from build123d import *

# Parameters (mm, degrees)
F2_R     = 2
F3_DEPTH = 1.1
F4_R     = 2.5
F5_DEPTH = 30


with BuildPart() as f1:
    # F0 (on Front) → F1 (revolve)
    with BuildSketch(Plane.XZ):
        Polygon((0, 1.9), (0, 0), (2.45, 1.9), align=None)
    revolve(axis=Axis((0, 0, 0.95), (0, 0, 1)))

    # F2 (on face) → F3 (join)
    with BuildSketch(Plane.XY.offset(1.9)):
        Circle(F2_R)
    extrude(amount=F3_DEPTH)

    # F4 (on face) → F5 (join)
    with BuildSketch(Plane.XY.offset(3)):
        with Locations((0, -0.214779)):
            Circle(F4_R)
    extrude(amount=F5_DEPTH)


solid = f1.part
The model under review builds one solid part; all positions refer to its coordinate system, in mm. A direction names the side the tool comes from. Give positions to 0.01 mm unless a question says otherwise; leave off trailing zeros. Write each loop counter-clockwise with the first axis right and the second up, starting at its lowest first coordinate (ties: lowest second). Pieces come first, ordered by that corner, then holes.
1. For P1, Ø1, axis at y = 1.5, z = 19, coming from the +X side (3 decimals); P2, Ø2, axis at x = 0, y = -1.5, coming from the -Z side, all flat-tipped, find the tip position at first contact; note any pin that passes through.
2. Tool access review of faces 1 (the cylindrical face through (-0.542, -2.655, 17.79)), 2 (the cylindrical face through (-0.434, -1.952, 2.442)): name each direction out of +Z, -Z, +X, -X, +Y, -Y from which nothing blocks a thin tool from reaching the whole face with its end or side.
3. Draft analysis for pull direction Z (two halves, no side actions). For faces 3 (the flat face through (1, -2, 3)), 4 (the conical face through (0, 0, 0)), 5 (the flat face through (0, 0, 33)), state which applies: +Z half, -Z half, draft (parallel to the pull), parting line (faces both ways), or undercut.
4. Wall thickness on L1, parallel to Z at x = -1.6, y = -1.55; L2, parallel to X at y = -0.7, z = 21.5; L3, parallel to X at y = 1.7, z = 11: over which ranges is each line inside the solid? List them lowest first.
5. Add section A-A, the plane z = 19. Write out the cut boundary in (x, y).
Worked answers:
1. P1: stops at x = 2.185
1. P2: stops at z = 0.39
2. face 1: +Z
2. face 2: none
3. face 3: undercut
3. face 4: -Z half
3. face 5: +Z half
4. L1: z = 1.73 to 1.9, 3 to 33
4. L2: x = -2.45 to 2.45
4. L3: x = -1.61 to 1.61
5. outline: circle Ø5 at (0, -0.21)
